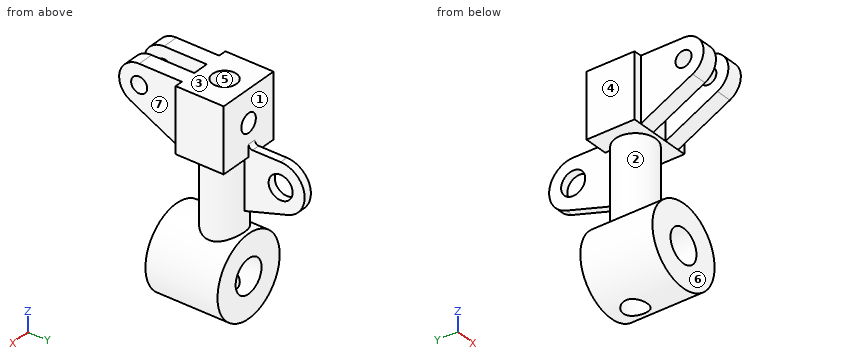
```python
from build123d import *

# Parameters (mm, degrees)
BOSS_EXTRUDE1_DEPTH       = 24
BOSS_EXTRUDE1_DEPTH_BACK  = 24
SKETCH1_W                 = 48
SKETCH1_H                 = 36
BOSS_EXTRUDE2_DEPTH       = 12
BOSS_EXTRUDE3_START       = -12
BOSS_EXTRUDE3_DEPTH       = 12
SKETCH7_R                 = 6
CUT_EXTRUDE1_DEPTH        = 105.675689632
SKETCH9_R                 = 30
SKETCH9_R_2               = 12.5
BOSS_EXTRUDE4_DEPTH       = 54
BOSS_EXTRUDE5_REACH       = 146.17
BOSS_EXTRUDE5_END_RADIUS  = 30
SKETCH10_R                = 15
SKETCH11_R                = 9
CUT_EXTRUDE2_DEPTH        = 185.480351361
BOSS_EXTRUDE6_START       = -87.205977382
BOSS_EXTRUDE6_DEPTH       = 39.205977382
BOSS_EXTRUDE6_START_2     = -77.335756752
BOSS_EXTRUDE6_2_DEPTH     = 29.335756752
BOSS_EXTRUDE6_START_3     = -6
BOSS_EXTRUDE6_3_OUTLINE_R = 9
BOSS_EXTRUDE6_3_DEPTH     = 6
CUT_EXTRUDE3_REACH        = 186.48
CUT_EXTRUDE3_END_RADIUS   = 9
SKETCH13_R                = 7


with BuildPart() as part:
    # Sketch1 → Boss-Extrude1 (new, two sides: drawn at the far end of the back side and taken through both)
    with BuildSketch(Plane(origin=(0, 0, 0), x_dir=(0, 0, -1), z_dir=(1, 0, 0)).offset(-BOSS_EXTRUDE1_DEPTH_BACK)):
        with Locations((24, -18)):
            Rectangle(SKETCH1_W, SKETCH1_H)
    extrude(amount=BOSS_EXTRUDE1_DEPTH + BOSS_EXTRUDE1_DEPTH_BACK)

    # Sketch2 → Boss-Extrude2 (add)
    with BuildSketch(Plane(origin=(18, 0, 0), x_dir=(0, 0, -1), z_dir=(1, 0, 0))):
        with BuildLine():
            Line((0, -36), (0, -68))
            ThreePointArc((0, -68), (11.519205494, -82.590547269), (28.384542614, -74.771559571))
            Line((28.384542614, -74.771559571), (48, -36))
            Line((48, -36), (0, -36))
        make_face()
    extrude(amount=-BOSS_EXTRUDE2_DEPTH)

    # Sketch6 → Boss-Extrude3 (add)
    with BuildSketch(Plane.ZY.offset(18).offset(BOSS_EXTRUDE3_START)):
        with BuildLine():
            Line((0, -36), (0, -68))
            ThreePointArc((0, -68), (-11.519205494, -82.590547269), (-28.384542614, -74.771559571))
            Line((-28.384542614, -74.771559571), (-48, -36))
            Line((-48, -36), (-48, 0))
            Line((-48, 0), (0, 0))
            Line((0, 0), (0, -36))
        make_face()
    extrude(amount=BOSS_EXTRUDE3_DEPTH)

    # Sketch7 → Cut-Extrude1 (cut, through all)
    with BuildSketch(Plane(origin=(18, 0, 0), x_dir=(0, 0, -1), z_dir=(1, 0, 0))):
        with Locations((15, -68)):
            Circle(SKETCH7_R)
    extrude(amount=-CUT_EXTRUDE1_DEPTH, mode=Mode.SUBTRACT)



with BuildPart() as body_2:
    # Sketch9 → Boss-Extrude4 (new body)
    with BuildSketch(Plane(origin=(0, 0, 0), x_dir=(1, 0, 0), z_dir=(0, 1, 0))):
        with Locations(Location((0, 132, 0), (0, 0, 270))):
            Circle(SKETCH9_R)
        with Locations(Location((0, 132, 0), (0, 0, 270))):
            Circle(SKETCH9_R_2, mode=Mode.SUBTRACT)
    extrude(amount=-BOSS_EXTRUDE4_DEPTH)


with BuildPart() as part_1:
    add(part.part)

    add(body_2.part)  # Boss-Extrude5 merges body 2
    # Boss-Extrude5: up to this cylinder (the profile starts outside it)
    boss_extrude5_end = Plane(origin=(0, -18.040976, -132), z_dir=(0, 1, 0)) * Cylinder(BOSS_EXTRUDE5_END_RADIUS, 353.34, mode=Mode.PRIVATE)
    # Sketch10 → Boss-Extrude5 (add, up to the surface)
    with BuildSketch(Plane(origin=(0, 0, -48), x_dir=(-1, 0, 0), z_dir=(0, 0, -1)), mode=Mode.PRIVATE) as boss_extrude5_sk1:
        with Locations(Location((0, -18.040976412, 0), (0, 0, 270))):
            Circle(SKETCH10_R)
    boss_extrude5_tool1 = extrude(boss_extrude5_sk1.sketch, amount=BOSS_EXTRUDE5_REACH, mode=Mode.PRIVATE) - boss_extrude5_end
    add(boss_extrude5_tool1.solids().sort_by_distance((0, -18.040976, -48))[0])

    # Sketch11 → Cut-Extrude2 (cut, through all)
    with BuildSketch(Plane.XY):
        with Locations((0, -18)):
            Circle(SKETCH11_R)
    extrude(amount=-CUT_EXTRUDE2_DEPTH, mode=Mode.SUBTRACT)

    # Boss-Extrude6: read off the stored shape, not the designer's step
    # Boss-Extrude6 outline → Boss-Extrude6 (add)
    with BuildSketch(Plane.XY.offset(BOSS_EXTRUDE6_START)):
        with BuildLine():
            ThreePointArc((8.763833852, -20.048222698), (4.591126901, -10.259098646), (-6, -11.291796068))
            Line((-6, -11.291796068), (-6, -20.048222698))
            Line((-6, -20.048222698), (8.763833852, -20.048222698))
        make_face()
    extrude(amount=BOSS_EXTRUDE6_DEPTH)

    # Boss-Extrude6 2 outline → Boss-Extrude6 2 (add)
    with BuildSketch(Plane.XY.offset(BOSS_EXTRUDE6_START_2)):
        with BuildLine():
            Line((0, 0), (-6, 0))
            Line((-6, 0), (-6, -4.293249327))
            ThreePointArc((-6, -4.293249327), (-3.064644655, -3.357381718), (0, -3.040976412))
            Line((0, -3.040976412), (0, 0))
        make_face()
    extrude(amount=BOSS_EXTRUDE6_2_DEPTH)

    # Boss-Extrude6 3 outline → Boss-Extrude6 3 (add)
    with BuildSketch(Plane.YZ.offset(BOSS_EXTRUDE6_START_3)):
        with BuildLine():
            Line((-6, -87.205977382), (-3.040976412, -87.205977382))
            Line((-3.040976412, -87.205977382), (29.319215471, -77.196102662))
            ThreePointArc((29.319215471, -77.196102662), (41.797890998, -57.310190334), (24, -42))
            Line((24, -42), (3, -42))
            ThreePointArc((3, -42), (0.878679656, -41.121320344), (0, -39))
            Line((0, -39), (0, -77.335756752))
            Line((0, -77.335756752), (-6, -77.335756752))
            Line((-6, -77.335756752), (-6, -87.205977382))
        make_face()
        with Locations((24, -60)):
            Circle(BOSS_EXTRUDE6_3_OUTLINE_R, mode=Mode.SUBTRACT)
    extrude(amount=BOSS_EXTRUDE6_3_DEPTH)

    # Cut-Extrude3: up to this cylinder (the profile starts outside it)
    cut_extrude3_end = Plane(origin=(0, -18, -24), z_dir=(0, 0, 1)) * Cylinder(CUT_EXTRUDE3_END_RADIUS, 391.96, mode=Mode.PRIVATE)
    # Sketch13 → Cut-Extrude3 (cut, up to the surface)
    with BuildSketch(Plane(origin=(0, 0, 0), x_dir=(1, 0, 0), z_dir=(0, 1, 0)), mode=Mode.PRIVATE) as cut_extrude3_sk1:
        with Locations(Location((0, 24, 0), (0, 0, 270))):
            Circle(SKETCH13_R)
    cut_extrude3_tool1 = extrude(cut_extrude3_sk1.sketch, amount=-CUT_EXTRUDE3_REACH, mode=Mode.PRIVATE) - cut_extrude3_end
    add(cut_extrude3_tool1.solids().sort_by_distance((0, 0, -24))[0], mode=Mode.SUBTRACT)


solid = part_1.part
```
Here's how the part is built. I have some questions about the finished solid (model axes, mm). Face numbers are marked on the shaded views. A direction names the side the tool comes from. Coordinates: 2 decimals unless noted, no trailing zeros. Order: outer loops, then holes, each group sorted by start corner. A loop starts at its lowest first (then second) coordinate and runs counter-clockwise, first axis right, second up.
1) We'd pull the mould along Z, two halves only. Please class the marked faces 1, 2 and 3: +Z half, -Z half, draft (parallel to the pull), parting line (faces both ways), or undercut.
2) Which directions (+Z, -Z, +X, -X, +Y, -Y) give clear straight access to the entire face, cutting with the end or side of a thin tool? Please do the marked faces 4, 5, 6 and 7.
3) Will these pins go through, and if not, where does the flat tip stop? pin 1 (8.5 mm diameter, centred on x = 0, z = -24, fed in from -Y); pin 2 (12 mm diameter, centred on x = 1.5, y = -15, fed in from +Z); pin 3 (3 mm diameter, centred on x = -4, y = 13.5, fed in from +Z); pin 4 (1 mm diameter, centred on x = -4, y = -3.5, fed in from -Z).
4) Imagine slicing it at D-D on z = -98.5. List the corners of the cut face in (x, y) for me, and give its area (3 significant figures).
5) I need wall thicknesses on line 1 (X direction, y = -75, z = -10); line 2 (X direction, y = -11, z = -132); line 3 (Y direction, x = 19, z = -113). Which ranges of each line are inside material? Lowest first, please.
6) Imagine slicing it at A-A on z = -15. List the corners of the cut face in (x, y) for me, and give its area (3 significant figures).
7) Imagine slicing it at B-B on z = -136. List the corners of the cut face in (x, y) for me, and give its area (3 significant figures).
8) Imagine slicing it at C-C on y = -45. List the corners of the cut face in (x, z) for me.
Response values:
1. face 1: draft
1. face 2: undercut
1. face 3: +Z half
2. face 4: +Z, -X, +Y, -Y
2. face 5: none
2. face 6: -Z, +X, -X, -Y
2. face 7: +Z, +X, -Y
3. pin 1: stops at y = -36
3. pin 2: stops at z = 0
3. pin 3: stops at z = -42
3. pin 4: stops at z = -161.8
4. outline: circle Ø30 at (0, -18.04); hole circle Ø18 at (0, -18)
4. area: 452 mm2
5. line 1: x = -18 to -6, 6 to 18
5. line 2: x = -30 to -12.5, 12.5 to 30
5. line 3: y = -54 to 0
6. outline: (-24, -36) - (-18, -36) - (-18, -62) - (-6, -62) - (-6, -36) - (6, -36) - (6, -62) - (18, -62) - (18, -36) - (24, -36) - (24, 0) - (-24, 0) - close; (-18, -83) - (-6, -83) - (-6, -74) - (-18, -74) - close; (6, -83) - (18, -83) - (18, -74) - (6, -74) - close; hole circle Ø18 at (0, -18)
6. area: 2,310 mm2
7. outline: (-29.73, -54) - (-11.84, -54) - (-11.84, 0) - (-29.73, 0) - close; (11.84, -54) - (29.73, -54) - (29.73, 0) - (11.84, 0) - close
7. area: 1,930 mm2
8. outline: circle Ø60 at (0, -132); (-18, -43.45) - (-6, -43.45) - (-6, 0) - (-18, 0) - close; (6, -43.45) - (18, -43.45) - (18, 0) - (6, 0) - close; hole circle Ø25 at (0, -132)
